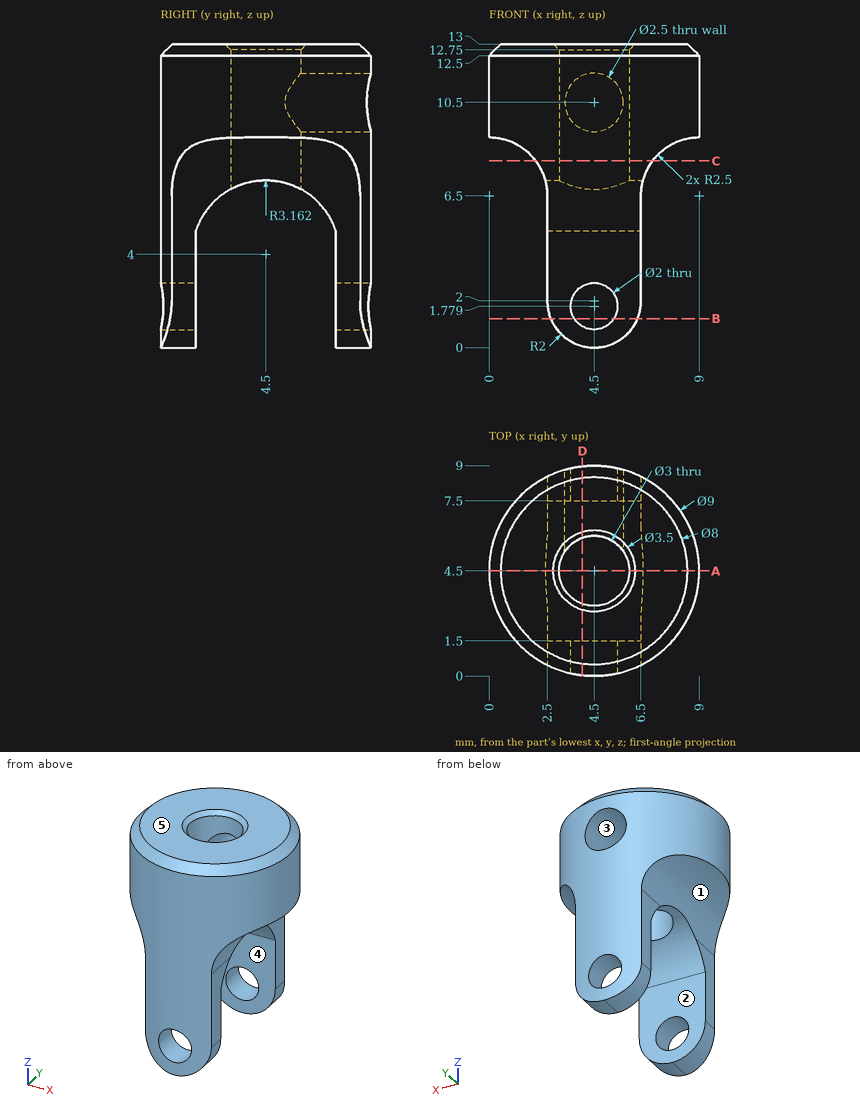
The drawing under review shows one solid part. Ordinate dimensions are in mm from its lowest x, y, z. A direction names the side the tool comes from. Round coordinates to 2 decimals unless told otherwise and drop trailing zeros. Write each loop counter-clockwise with the first axis right and the second up, starting at its lowest first coordinate (ties: lowest second). Pieces come first, ordered by that corner, then holes. Notation, with made-up numbers: (17, 24) - (27, 24) arc R24 ccw to (27, 54) - close; hole circle Ø6 at (29.25, 42). An arc over 180 degrees is marked (long way). Put each result on its own line as item: value.
Q1. We need section C-C (z = 8). Give the boundary of the cut face in (x, y), and give its area (3 significant figures).
Solved:
outline: (2, 0.76) arc R4.5 ccw to (7, 0.76) - (7, 8.24) arc R4.5 ccw to (2, 8.24) - close; hole circle Ø3 at (4.5, 4.5)
area: 35.5 mm2
Q2. We need section D-D (x = 4). Count the separate pieces of the cut face and the enclosed holes in it.
Solved:
separate pieces: 5
enclosed holes: 0
Q3. Wall thickness on probe 1 along Y at (x, z) = (3, 1.5); probe 2 along X at (y, z) = (6.5, 12); probe 3 along X at (y, z) = (3.5, 12.25): over which ranges is each line inside the solid? List them lowest first.
Solved:
probe 1: y = 0.26 to 1.5, 7.5 to 8.74
probe 2: x = 0.47 to 8.53
probe 3: x = 0.11 to 3.38, 5.62 to 8.89
Q4. Machinability: for the marked faces 1 and 2, which of the approach directions +Z, -Z, +X, -X, +Y, -Y give a long, thin tool a straight path to every point of the face, cutting with its end or side? Answer none if there is none.
Solved:
face 1: -Z, -X, +Y, -Y
face 2: -Z, +X, -X
Q5. We need section A-A (y = 4.5). Give the boundary of the cut face in (x, z).
Solved:
outline: (0, 9) arc R2.5 cw to (2.41, 7.16) - (3, 7.16) - (3, 12.75) - (2.75, 13) - (0.5, 13) - (0, 12.5) - close; (6, 7.16) - (6.59, 7.16) arc R2.5 cw to (9, 9) - (9, 12.5) - (8.5, 13) - (6.25, 13) - (6, 12.75) - close
Q6. Insertion check: pin 1 Ø2 at (x, z) = (4.5, 1.5) entering from +Y; pin 2 Ø2.5 at (y, z) = (7.5, 4.5) entering from -X; pin 3 Ø3 at (x, y) = (2.5, 4.5) entering from -Z; pin 4 Ø2 at (x, z) = (4.5, 10.5) entering from +Y. Each pin has a flat end and moves straight along its axis. Give the tip position at first contact, or say it passes through.
Solved:
pin 1: stops at y = 9
pin 2: stops at x = 2.5
pin 3: stops at z = 6.78
pin 4: stops at y = 3.38
Q7. We need section B-B (z = 1.25). Give the boundary of the cut face in (x, y).
Solved:
outline: (2.65, 0.4) arc R4.5 ccw to (3.65, 0.08) - (3.65, 1.5) - (2.65, 1.5) - close; (2.65, 7.5) - (3.65, 7.5) - (3.65, 8.92) arc R4.5 ccw to (2.65, 8.6) - close; (5.35, 0.08) arc R4.5 ccw to (6.35, 0.4) - (6.35, 1.5) - (5.35, 1.5) - close; (5.35, 7.5) - (6.35, 7.5) - (6.35, 8.6) arc R4.5 ccw to (5.35, 8.92) - close
Q8. Mouldability with a two-part tool opening along Z and no side actions: class the marked faces 3, 4 and 5 as released by +Z, released by -Z, zero draft, split by the parting line, or undercut.
Solved:
face 3: undercut
face 4: zero draft
face 5: released by +Z
